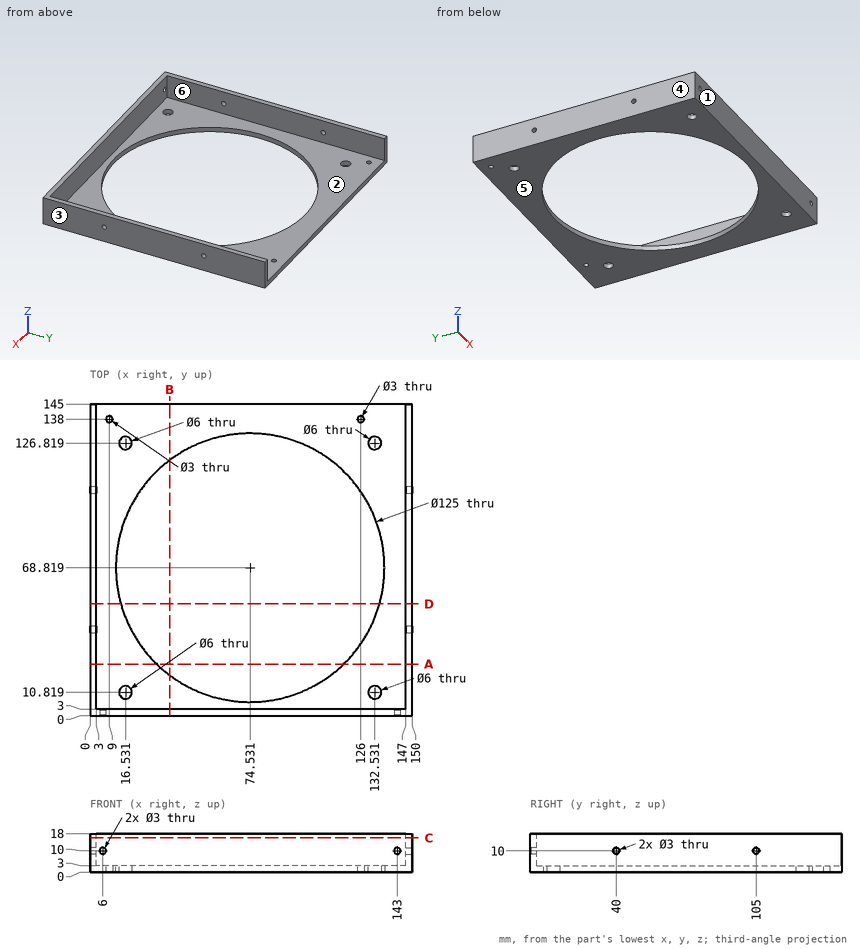
Source: three-view drawing plus pictorial views. Frame: mm from the lowest corner of the part. A direction names the side the tool comes from. Round coordinates to 2 decimals unless told otherwise and drop trailing zeros. Loops run counter-clockwise (first coordinate to the right, second up) from the corner with the lowest first, then second, coordinate; pieces in that order, holes last. Notation, with made-up numbers: M 10,-7 L 39,-7 A24 cw 39,20 Z; hole C 77,19 d6. An arc over 180 degrees is marked long. Answer as CSV lines item,"result". Start each with the question number.
(1) Section A-A, the plane y = 24. Output: boundary loops of the cut face in (x, z).
(2) Section D-D, the plane y = 52. Output: boundary loops of the cut face in (x, z).
(3) Line query: line 1 (X direction, y = 138, z = 2.2); line 2 (X direction, y = 57.5, z = 17.25); line 3 (Z direction, x = 149, y = 105). Output: solid intervals per line, ascending. Write a range as [from, to].
(4) Section B-B, the plane x = 37. Output: boundary loops of the cut face in (y, z) (1 decimal).
(5) Draft query along X for the marked faces 3, 4, 5 and 6. Return one class per face: released by +X, released by -X, zero draft, split by the parting line, or undercut.
(6) Reachability of the marked faces 1 and 2 from +Z, -Z, +X, -X, +Y, -Y: full face, straight path, thin tool, end or side. Return the list, or none.
(7) First-contact query: pin 1 (4 mm diameter, centred on x = 6, z = 10, fed in from -Y); pin 2 (4 mm diameter, centred on x = 110, z = 5.5, fed in from +Y); pin 3 (8 mm diameter, centred on x = 16.53, y = 126.82, fed in from +Z). Flat tips, straight axial feed; report the tip coordinate or a pass-through.
(8) Section C-C, the plane z = 16. Output: boundary loops of the cut face in (x, y), plus the area to 3 significant figures.
Values found:
1,outline,"M 0,0 L 30.97,0 L 30.97,3 L 3,3 L 3,18 L 0,18 Z; M 118.09,0 L 150,0 L 150,18 L 147,18 L 147,3 L 118.09,3 Z"
2,outline,"M 0,0 L 14.34,0 L 14.34,3 L 3,3 L 3,18 L 0,18 Z; M 134.73,0 L 150,0 L 150,18 L 147,18 L 147,3 L 134.73,3 Z"
3,line 1,"x = [0, 7.5], [10.5, 124.5], [127.5, 150]"
3,line 2,"x = [0, 3], [147, 150]"
3,line 3,"z = [0, 8.5], [11.5, 18]"
4,outline,"M 0,0 L 18.8,0 L 18.8,3 L 3,3 L 3,18 L 0,18 Z; M 118.8,0 L 145,0 L 145,3 L 118.8,3 Z"
5,face 3,"released by +X"
5,face 4,"released by -X"
5,face 5,"zero draft"
5,face 6,"undercut"
6,face 1,"+Z, -Z, +X, -X, -Y"
6,face 2,"+Z, +Y"
7,pin 1,"stops at y = 0"
7,pin 2,"stops at y = 3"
7,pin 3,"stops at z = 3"
8,outline,"M 0,0 L 150,0 L 150,145 L 147,145 L 147,3 L 3,3 L 3,145 L 0,145 Z"
8,area,"1,300 mm²"
